Source: three-view drawing plus pictorial views. Frame: mm from the lowest corner of the part. A direction names the side the tool comes from. Give positions to 0.01 mm unless a question says otherwise; leave off trailing zeros. Write each loop counter-clockwise with the first axis right and the second up, starting at its lowest first coordinate (ties: lowest second). Pieces come first, ordered by that corner, then holes.
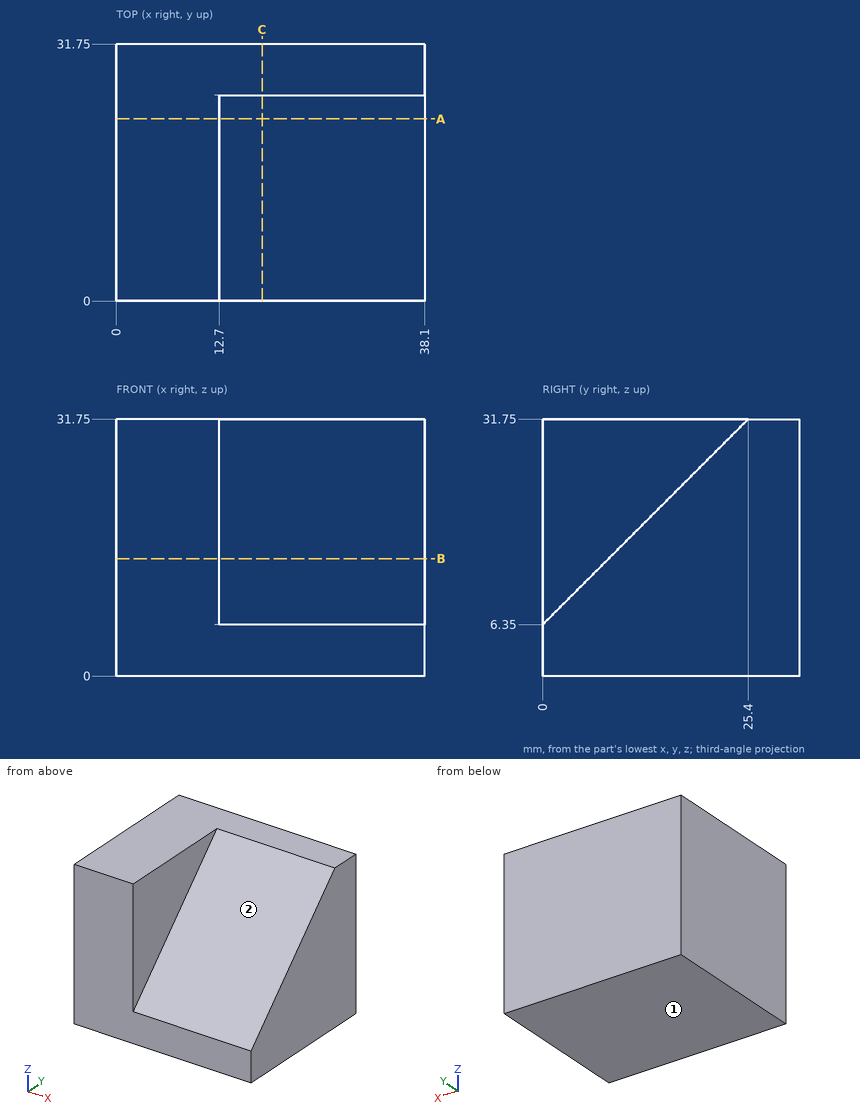
Q1. Access query for the marked faces 1 and 2. Directions: +Z, -Z, +X, -X, +Y, -Y. A direction counts if a zero-diameter tool reaches every point of the face in a straight line with its end or side. Return the directions, or none.
Filled sheet:
face 1: -Z, +X, -X, +Y, -Y
face 2: +Z, +X, -Y
Q2. Section A-A on y = 22.5. Output: boundary loops of the cut face in (x, z).
Filled sheet:
outline: (0, 0) - (38.1, 0) - (38.1, 28.85) - (12.7, 28.85) - (12.7, 31.75) - (0, 31.75) - close
Q3. Ray query, line 1 along X through (y, z) = (17, 25); line 2 along Z through (x, y) = (34.5, 22); line 3 along Z through (x, y) = (25, 15.5). Return the intervals inside material, ascending.
Filled sheet:
line 1: x = 0 to 12.7
line 2: z = 0 to 28.35
line 3: z = 0 to 21.85
Q4. Pin query (flat end, axial travel): P1, Ø3, axis at x = 25.5, z = 13, coming from the -Y side; P2, Ø5, axis at x = 29, z = 17, coming from the -Y side; P3, Ø2, axis at x = 30, z = 19, coming from the -Y side. Return the tip coordinate at first contact, or that it passes through.
Filled sheet:
P1: stops at y = 5.15
P2: stops at y = 8.15
P3: stops at y = 11.65
Q5. Section B-B on z = 14.5. Output: boundary loops of the cut face in (x, y), plus the area to 3 significant figures.
Filled sheet:
outline: (0, 0) - (12.7, 0) - (12.7, 8.15) - (38.1, 8.15) - (38.1, 31.75) - (0, 31.75) - close
area: 1,000 mm2
Q6. Section C-C on x = 18. Output: boundary loops of the cut face in (y, z).
Filled sheet:
outline: (0, 0) - (31.75, 0) - (31.75, 31.75) - (25.4, 31.75) - (0, 6.35) - close
